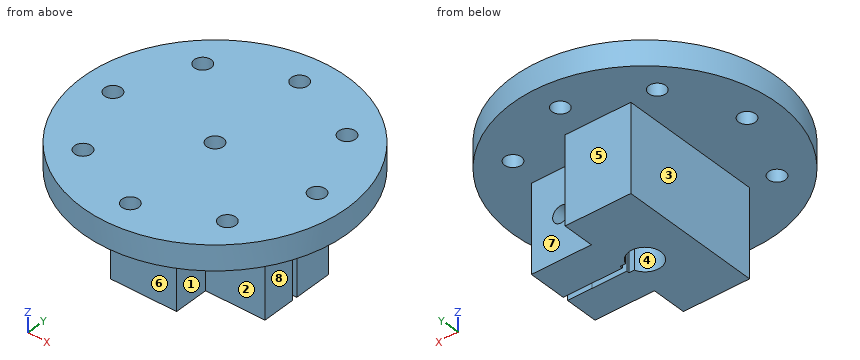
```python
from build123d import *

# Parameters (mm, degrees)
SKETCH_1_W           = 30
SKETCH_1_H           = 14.828427124
EXTRUDE_2_DEPTH      = 33
CUT_EXTRUDE_9_DEPTH  = 46
CUT_EXTRUDE_10_DEPTH = 30
CUT_EXTRUDE_12_DEPTH = 40
CUT_EXTRUDE_13_DEPTH = 46
CUT_EXTRUDE_18_DEPTH = 285
SKETCH_12_R          = 50
EXTRUDE_7_DEPTH      = 9.398
SKETCH_12_5_R        = 3.175
CUT_EXTRUDE_27_DEPTH = 63
SKETCH_20_R          = 6
SKETCH_20_R_2        = 3.175
EXTRUDE_9_DEPTH      = 3
CUT_EXTRUDE_29_DEPTH = 31
CUT_EXTRUDE_30_DEPTH = 33
CUT_EXTRUDE_31_DEPTH = 33
CUT_EXTRUDE_32_DEPTH = 33
SKETCH_21_R          = 6
SKETCH_21_R_2        = 3.175
EXTRUDE_11_DEPTH     = 34
SKETCH_21_5_R        = 6
SKETCH_21_5_R_2      = 3.175
CUT_EXTRUDE_34_DEPTH = 31
SKETCH_22_R          = 3.175
CUT_EXTRUDE_35_DEPTH = 31
SKETCH_24_W          = 25
SKETCH_24_H          = 20
EXTRUDE_12_DEPTH     = 33
SKETCH_24_3_W        = 9.986704705
SKETCH_24_3_H        = 14.062123622
EXTRUDE_13_DEPTH     = 34
SKETCH_25_W          = 9.1968428
SKETCH_25_H          = 2
EXTRUDE_14_DEPTH     = 33
EXTRUDE_15_DEPTH     = 36
SKETCH_28_W          = 22.632732516
SKETCH_28_H          = 2.5
SKETCH_28_W_2        = 22.447864345
CUT_EXTRUDE_43_DEPTH = 33
SKETCH_1_32_W        = 0.7
SKETCH_1_32_H        = 1
CUT_EXTRUDE_45_DEPTH = 33
SKETCH_27_R          = 3.175
CUT_EXTRUDE_46_DEPTH = 70


with BuildPart() as part:
    # Sketch 1 → Extrude 2 (new body)
    with BuildSketch(Plane.XY):
        with Locations((7.585786438, 0)):
            Rectangle(SKETCH_1_W, SKETCH_1_H)
    extrude(amount=EXTRUDE_2_DEPTH)

    # Sketch 1_11 → Cut-Extrude 9 (cut)
    with BuildSketch(Plane.XY):
        with BuildLine():
            Line((0, -2), (0, 0))
            Line((0, 0), (-6, 0))
            ThreePointArc((-6, 0), (-4.242640687, -4.242640687), (0, -6))
            ThreePointArc((0, -6), (3.464101615, -4.898979486), (5.656854249, -2))
            Line((5.656854249, -2), (0, -2))
        make_face()
    extrude(amount=CUT_EXTRUDE_9_DEPTH, mode=Mode.SUBTRACT)

    # Sketch 1_12 → Cut-Extrude 10 (cut)
    with BuildSketch(Plane.XY):
        with BuildLine():
            Line((-6, 0), (0, 0))
            Line((0, 0), (0, 2))
            Line((0, 2), (0, 6))
            ThreePointArc((0, 6), (-4.242640687, 4.242640687), (-6, 0))
        make_face()
    extrude(amount=CUT_EXTRUDE_10_DEPTH, mode=Mode.SUBTRACT)

    # Sketch 1_14 → Cut-Extrude 12 (cut)
    with BuildSketch(Plane.XY):
        with BuildLine():
            Line((6, 0), (0, 0))
            Line((0, 0), (0, -2))
            Line((0, -2), (5.656854249, -2))
            ThreePointArc((5.656854249, -2), (5.913591358, -1.014611872), (6, 0))
        make_face()
    extrude(amount=CUT_EXTRUDE_12_DEPTH, mode=Mode.SUBTRACT)

    # Sketch 1_15 → Cut-Extrude 13 (cut)
    with BuildSketch(Plane.XY):
        with BuildLine():
            Line((0, 6), (0, 2))
            Line((0, 2), (5.656854249, 2))
            ThreePointArc((5.656854249, 2), (3.464101615, 4.898979486), (0, 6))
        make_face()
    extrude(amount=CUT_EXTRUDE_13_DEPTH, mode=Mode.SUBTRACT)

    # Sketch 1_20 → Cut-Extrude 18 (cut)
    with BuildSketch(Plane.XY):
        with BuildLine():
            ThreePointArc((7.414213562, 7.414213562), (9.005239827, 5.370919954), (10.046946078, 3))
            Line((10.046946078, 3), (18, 3))
            Line((18, 3), (20.850103278, 3))
            Line((20.850103278, 3), (20.850103278, 1))
            Line((20.850103278, 1), (18, 1))
            Line((18, 1), (18, -1))
            Line((18, -1), (20.850103278, -1))
            Line((20.850103278, -1), (20.850103278, -3))
            Line((20.850103278, -3), (18, -3))
            Line((18, -3), (10.046946078, -3))
            ThreePointArc((10.046946078, -3), (9.005239827, -5.370919954), (7.414213562, -7.414213562))
            Line((7.414213562, -7.414213562), (22.585786438, -7.414213562))
            Line((22.585786438, -7.414213562), (22.585786438, 7.414213562))
            Line((22.585786438, 7.414213562), (7.414213562, 7.414213562))
        make_face()
    extrude(amount=CUT_EXTRUDE_18_DEPTH, mode=Mode.SUBTRACT)

    # Sketch 12 → Extrude 7 (add)
    with BuildSketch(Plane.XY.offset(33)):
        Circle(SKETCH_12_R)
    extrude(amount=EXTRUDE_7_DEPTH)

    # Sketch 12_5 → Cut-Extrude 27 (cut)
    with BuildSketch(Plane.XY.offset(33)):
        with Locations((27.24506403, 27.24506403)):
            Circle(SKETCH_12_5_R)
        with Locations((-27.24506403, 27.24506403)):
            Circle(SKETCH_12_5_R)
        with Locations((-38.530339059, 0)):
            Circle(SKETCH_12_5_R)
        with Locations((-27.24506403, -27.24506403)):
            Circle(SKETCH_12_5_R)
        with Locations((0, -38.530339059)):
            Circle(SKETCH_12_5_R)
        with Locations((27.24506403, -27.24506403)):
            Circle(SKETCH_12_5_R)
        with Locations((38.530339059, 0)):
            Circle(SKETCH_12_5_R)
        with Locations((0, 38.530339059)):
            Circle(SKETCH_12_5_R)
    extrude(amount=CUT_EXTRUDE_27_DEPTH, mode=Mode.SUBTRACT)

    # Sketch 20 → Extrude 9 (add)
    with BuildSketch(Plane(origin=(0, 0, 0), x_dir=(-1, 0, 0), z_dir=(0, 0, -1))):
        Circle(SKETCH_20_R)
        Circle(SKETCH_20_R_2, mode=Mode.SUBTRACT)
    extrude(amount=-EXTRUDE_9_DEPTH)

    # Sketch 1_26 → Cut-Extrude 29 (cut)
    with BuildSketch(Plane.XY):
        with BuildLine():
            ThreePointArc((10.485281374, 0), (10.473325852, -0.500570761), (10.437486551, -1))
            Line((10.437486551, -1), (18, -1))
            Line((18, -1), (18, 1))
            Line((18, 1), (10.437486551, 1))
            ThreePointArc((10.437486551, 1), (10.473325852, 0.500570761), (10.485281374, 0))
        make_face()
        with BuildLine():
            Line((7, 1), (7, 0))
            Line((7, 0), (7, -1))
            Line((7, -1), (7.7, -1))
            Line((7.7, -1), (10.437486551, -1))
            ThreePointArc((10.437486551, -1), (10.473325852, -0.500570761), (10.485281374, 0))
            ThreePointArc((10.485281374, 0), (10.473325852, 0.500570761), (10.437486551, 1))
            Line((10.437486551, 1), (7.7, 1))
            Line((7.7, 1), (7, 1))
        make_face()
    extrude(amount=CUT_EXTRUDE_29_DEPTH, mode=Mode.SUBTRACT)

    # Sketch 1_27 → Cut-Extrude 30 (cut)
    with BuildSketch(Plane.XY):
        with BuildLine():
            Line((0, 2), (0, 0))
            Line((0, 0), (6, 0))
            ThreePointArc((6, 0), (5.913591358, 1.014611872), (5.656854249, 2))
            Line((5.656854249, 2), (0, 2))
        make_face()
        with BuildLine():
            ThreePointArc((10.485281374, 0), (10.473325852, -0.500570761), (10.437486551, -1))
            Line((10.437486551, -1), (18, -1))
            Line((18, -1), (18, 1))
            Line((18, 1), (10.437486551, 1))
            ThreePointArc((10.437486551, 1), (10.473325852, 0.500570761), (10.485281374, 0))
        make_face()
        with BuildLine():
            Line((7, 1), (7, 0))
            Line((7, 0), (7, -1))
            Line((7, -1), (7.7, -1))
            Line((7.7, -1), (10.437486551, -1))
            ThreePointArc((10.437486551, -1), (10.473325852, -0.500570761), (10.485281374, 0))
            ThreePointArc((10.485281374, 0), (10.473325852, 0.500570761), (10.437486551, 1))
            Line((10.437486551, 1), (7.7, 1))
            Line((7.7, 1), (7, 1))
        make_face()
    extrude(amount=CUT_EXTRUDE_30_DEPTH, mode=Mode.SUBTRACT)

    # Sketch 1_28 → Cut-Extrude 31 (cut)
    with BuildSketch(Plane.XY):
        with BuildLine():
            Line((-6, 0), (0, 0))
            Line((0, 0), (0, 2))
            Line((0, 2), (0, 6))
            ThreePointArc((0, 6), (-4.242640687, 4.242640687), (-6, 0))
        make_face()
        with BuildLine():
            Line((6, 0), (0, 0))
            Line((0, 0), (0, -2))
            Line((0, -2), (5.656854249, -2))
            ThreePointArc((5.656854249, -2), (5.913591358, -1.014611872), (6, 0))
        make_face()
        with BuildLine():
            Line((6, -2), (6, 0))
            ThreePointArc((6, 0), (5.913591358, -1.014611872), (5.656854249, -2))
            Line((5.656854249, -2), (6, -2))
        make_face()
        with BuildLine():
            ThreePointArc((5.656854249, 2), (5.913591358, 1.014611872), (6, 0))
            Line((6, 0), (6, 2))
            Line((6, 2), (5.656854249, 2))
        make_face()
        Polygon((6, 2), (6, 0), (7, 0), (7, 1), (7, 2), align=None)
        Polygon((7, 0), (6, 0), (6, -2), (7, -2), (7, -1), align=None)
    extrude(amount=CUT_EXTRUDE_31_DEPTH, mode=Mode.SUBTRACT)

    # Sketch 1_29 → Cut-Extrude 32 (cut)
    with BuildSketch(Plane.XY):
        with BuildLine():
            Line((0, 6), (0, 2))
            Line((0, 2), (5.656854249, 2))
            ThreePointArc((5.656854249, 2), (3.464101615, 4.898979486), (0, 6))
        make_face()
        with BuildLine():
            Line((0, -2), (0, 0))
            Line((0, 0), (-6, 0))
            ThreePointArc((-6, 0), (-4.242640687, -4.242640687), (0, -6))
            ThreePointArc((0, -6), (3.464101615, -4.898979486), (5.656854249, -2))
            Line((5.656854249, -2), (0, -2))
        make_face()
    extrude(amount=CUT_EXTRUDE_32_DEPTH, mode=Mode.SUBTRACT)

    # Sketch 21 → Extrude 11 (add)
    with BuildSketch(Plane(origin=(0, 0, 0), x_dir=(-1, 0, 0), z_dir=(0, 0, -1))):
        Circle(SKETCH_21_R)
        Circle(SKETCH_21_R_2, mode=Mode.SUBTRACT)
    extrude(amount=-EXTRUDE_11_DEPTH)

    # Sketch 21_5 → Cut-Extrude 34 (cut)
    with BuildSketch(Plane(origin=(0, 0, 0), x_dir=(-1, 0, 0), z_dir=(0, 0, -1))):
        Circle(SKETCH_21_5_R)
        Circle(SKETCH_21_5_R_2, mode=Mode.SUBTRACT)
    extrude(amount=-CUT_EXTRUDE_34_DEPTH, mode=Mode.SUBTRACT)

    # Sketch 22 → Cut-Extrude 35 (cut)
    with BuildSketch(Plane(origin=(0, 0, 33), x_dir=(-1, 0, 0), z_dir=(0, 0, -1))):
        Circle(SKETCH_22_R)
    extrude(amount=-CUT_EXTRUDE_35_DEPTH, mode=Mode.SUBTRACT)

    # Sketch 24 → Extrude 12 (add)
    with BuildSketch(Plane(origin=(0, 0, 0), x_dir=(-1, 0, 0), z_dir=(0, 0, -1))):
        with Locations((4.900918267, -16.64791006)):
            Rectangle(SKETCH_24_W, SKETCH_24_H)
    extrude(amount=-EXTRUDE_12_DEPTH)

    # Sketch 24_3 → Extrude 13 (add)
    with BuildSketch(Plane(origin=(0, 0, 0), x_dir=(-1, 0, 0), z_dir=(0, 0, -1))):
        with Locations((12.407565915, 0.383151751)):
            Rectangle(SKETCH_24_3_W, SKETCH_24_3_H)
        Polygon((-7.414213562, 27.414213562), (-7.414213562, 7.414213562), (7.414213562, 7.414213562), (17.400918267, 7.414213562), (17.400918267, 27.414213562), align=None)
    extrude(amount=-EXTRUDE_13_DEPTH)

    # Sketch 25 → Extrude 14 (add)
    with BuildSketch(Plane(origin=(0, 0, 0), x_dir=(-1, 0, 0), z_dir=(0, 0, -1))):
        Polygon((-20.850103278, -1), (-20.850103278, -0.961195415), (-30.046946078, -0.961195415), (-30.046946078, -3), (-20.850103278, -3), align=None)
        with Locations((-25.448524678, 2)):
            Rectangle(SKETCH_25_W, SKETCH_25_H)
    extrude(amount=-EXTRUDE_14_DEPTH)

    # Sketch 26 → Extrude 15 (add)
    with BuildSketch(Plane(origin=(0, 0, 0), x_dir=(-1, 0, 0), z_dir=(0, 0, -1))):
        with BuildLine():
            Line((-30.046946078, 18), (-30.046946078, 3))
            Line((-30.046946078, 3), (-10.046946078, 3))
            ThreePointArc((-10.046946078, 3), (-9.005239827, 5.370919954), (-7.414213562, 7.414213562))
            Line((-7.414213562, 7.414213562), (-7.414213562, 18))
            Line((-7.414213562, 18), (-30.046946078, 18))
        make_face()
        with BuildLine():
            Line((-10.046946078, -3), (-30.046946078, -3))
            Line((-30.046946078, -3), (-30.046946078, -15.961195415))
            Line((-30.046946078, -15.961195415), (-7.599081733, -15.961195415))
            Line((-7.599081733, -15.961195415), (-7.599081733, -7.224616412))
            ThreePointArc((-7.599081733, -7.224616412), (-9.072343707, -5.256777069), (-10.046946078, -3))
        make_face()
    extrude(amount=-EXTRUDE_15_DEPTH)

    # Sketch 28 → Cut-Extrude 43 (cut)
    with BuildSketch(Plane(origin=(0, 0, 0), x_dir=(-1, 0, 0), z_dir=(0, 0, -1))):
        with Locations((-18.73057982, 16.75)):
            Rectangle(SKETCH_28_W, SKETCH_28_H)
        with Locations((-18.823013906, -14.711195415)):
            Rectangle(SKETCH_28_W_2, SKETCH_28_H)
    extrude(amount=-CUT_EXTRUDE_43_DEPTH, mode=Mode.SUBTRACT)

    # Sketch 1_32 → Cut-Extrude 45 (cut)
    with BuildSketch(Plane.XY):
        with Locations((7.35, 1.5)):
            Rectangle(SKETCH_1_32_W, SKETCH_1_32_H)
        with Locations((7.35, -1.5)):
            Rectangle(SKETCH_1_32_W, SKETCH_1_32_H)
    extrude(amount=CUT_EXTRUDE_45_DEPTH, mode=Mode.SUBTRACT)

    # Sketch 27 → Cut-Extrude 46 (cut)
    with BuildSketch(Plane.XZ.offset(15.961195415)):
        with Locations((18.823013906, 16.5)):
            Circle(SKETCH_27_R)
    extrude(amount=-CUT_EXTRUDE_46_DEPTH, mode=Mode.SUBTRACT)


solid = part.part
```
Could you check a few things on this model? Use its own coordinates, in mm. Face numbers are marked on the shaded views. A direction names the side the tool comes from. Round coordinates to 2 decimals unless told otherwise and drop trailing zeros. Loops run counter-clockwise (first coordinate to the right, second up) from the corner with the lowest first, then second, coordinate; pieces in that order, holes last. Notation, with made-up numbers: (56, 59) - (90, 59) arc R26 cw to (90, 90) - close; hole circle Ø3 at (-38.5, -33). An arc over 180 degrees is marked (long way). Use CSV: the item, a comma, the result in double quotes.
Item 1: If we section it at B-B on z = 16.5: List the corners of the cut face in (x, y) for me, then the cut area to 3 significant figures.
Here are the results:
outline,"(-17.4, -26.65) - (7.6, -26.65) - (7.6, -13.46) - (15.65, -13.46) - (15.65, -1) - (7.7, -1) - (7.7, -2) - (5.66, -2) arc R6 cw (long way) to (5.66, 2) - (7.7, 2) - (7.7, 1) - (15.65, 1) - (15.65, 15.5) - (7.41, 15.5) - (7.41, 27.41) - (-17.4, 27.41) - close; (22, -13.46) - (30.05, -13.46) - (30.05, -0.96) - (22, -0.96) - close; (22, 1) - (30.05, 1) - (30.05, 15.5) - (22, 15.5) - close"
area,"1,660 mm²"
Item 2: For the marked faces 5, 6, 7 and 8, which set-ups out of +Z, -Z, +X, -X, +Y, -Y let a thin tool reach every point of the face, with its end or its side?
Here are the results:
face 5,"-Z, +X, -X, +Y"
face 6,"-Z, +X, -X, -Y"
face 7,"-Z, +X, +Y"
face 8,"-Z, +X, +Y, -Y"
Item 3: If we section it at A-A on x = 0: List the corners of the cut face in (y, z) for me (3 decimals).
Here are the results:
outline,"(-50, 33) - (-41.705, 33) - (-41.705, 42.398) - (-50, 42.398) - close; (-35.355, 33) - (-26.648, 33) - (-26.648, 0) - (-6, 0) - (-6, 31) - (-3.175, 31) - (-3.175, 42.398) - (-35.355, 42.398) - close; (3.175, 31) - (6, 31) - (6, 0) - (27.414, 0) - (27.414, 33) - (35.355, 33) - (35.355, 42.398) - (3.175, 42.398) - close; (41.705, 33) - (50, 33) - (50, 42.398) - (41.705, 42.398) - close"
Item 4: If we section it at C-C on y = 40.5: List the corners of the cut face in (x, z) for me.
Here are the results:
outline,"(-29.32, 33) - (-2.49, 33) - (-2.49, 42.4) - (-29.32, 42.4) - close; (2.49, 33) - (29.32, 33) - (29.32, 42.4) - (2.49, 42.4) - close"
Item 5: I need wall thicknesses on L1, parallel to Y at x = 0, z = 36.75 (3 decimals); L2, parallel to Z at x = 21.5, y = -22.5; L3, parallel to X at y = -26.5, z = 10. Which ranges of each line are inside material? Lowest first, please. Write a range as [from, to].
Here are the results:
L1,"y = [-50, -41.705], [-35.355, -3.175], [3.175, 35.355], [41.705, 50]"
L2,"z = [33, 42.4]"
L3,"x = [-17.4, 7.6]"
Item 6: Will these pins go through, and if not, where does the flat tip stop? pin 1 (4 mm diameter, centred on x = 25.5, z = 35, fed in from -Y); pin 2 (14 mm diameter, centred on y = -9, z = 13, fed in from +X); pin 3 (10 mm diameter, centred on y = 20, z = 17, fed in from -X).
Here are the results:
pin 1,"stops at y = -44.13"
pin 2,"stops at x = 30.05"
pin 3,"stops at x = -17.4"
Item 7: If we mould it in two halves opening along X, with no side actions, what happens to the marked faces 1, 2, 3 and 4? For each: pulls with the +X half, pulls with the -X half, needs draft (parallel to the pull), parting line crosses it, or undercut.
Here are the results:
face 1,"pulls with the +X half"
face 2,"needs draft"
face 3,"pulls with the -X half"
face 4,"undercut"
Item 8: If we section it at D-D on z = 40: Count the separate pieces of the cut face and the enclosed holes in it, then the cut area to 3 significant figures.
Here are the results:
separate pieces,"1"
enclosed holes,"9"
area,"7,570 mm²"
